```python
from build123d import *

# Parameters (mm, degrees)
SKETCH1_W                 = 2.116666666
SKETCH1_H                 = 3.175
SKETCH1_W_2               = 3.175
SKETCH1_H_2               = 2.116666666
SKETCH1_W_3               = 6.35
SKETCH1_H_3               = 37.666666667
SKETCH1_W_4               = 33.666666667
SKETCH1_H_4               = 6.35
BOSS_EXTRUDE1_DEPTH       = 3.175
SKETCH3_W                 = 3.175
SKETCH3_H                 = 3.175
SKETCH3_W_2               = 97.825
SKETCH3_H_2               = 109.825
BOSS_EXTRUDE2_DEPTH       = 3.175
MIRROR5_COPY_1_SKETCH_W   = 2.116666666
MIRROR5_COPY_1_SKETCH_H   = 3.175
MIRROR5_COPY_1_SKETCH_W_2 = 3.175
MIRROR5_COPY_1_SKETCH_H_2 = 2.116666666
MIRROR5_COPY_1_SKETCH_W_3 = 6.35
MIRROR5_COPY_1_SKETCH_H_3 = 37.666666667
MIRROR5_COPY_1_SKETCH_W_4 = 33.666666667
MIRROR5_COPY_1_SKETCH_H_4 = 6.35
MIRROR5_COPY_1_DEPTH      = 3.175
MIRROR5_COPY_2_SKETCH_W   = 3.175
MIRROR5_COPY_2_SKETCH_H   = 3.175
MIRROR5_COPY_2_SKETCH_W_2 = 97.825
MIRROR5_COPY_2_SKETCH_H_2 = 109.825
MIRROR5_COPY_2_DEPTH      = 3.175


with BuildPart() as part:
    # Sketch1 → Boss-Extrude1 (new body)
    # profile 1 of 4: a face of its own
    with BuildSketch(Plane(origin=(0, 0, 0), x_dir=(1, 0, 0), z_dir=(0, 1, 0))):
        Polygon((0, 122.525), (0, 135.225), (-123.225, 135.225), (-123.225, 0), (-110.525, 0), (-110.525, 37.666666667), (-110.525, 40.841666667), (-110.525, 122.525), (-78.927699489, 122.525), (-36.841666667, 122.525), (-33.666666667, 122.525), align=None)
        with Locations((-113.7, 39.254166667)):
            Rectangle(SKETCH1_W, SKETCH1_H, mode=Mode.SUBTRACT)
        with Locations((-35.254166667, 125.7)):
            Rectangle(SKETCH1_W_2, SKETCH1_H_2, mode=Mode.SUBTRACT)
    # profile 2 of 4: a face of its own
    with BuildSketch(Plane(origin=(0, 0, 0), x_dir=(1, 0, 0), z_dir=(0, 1, 0))):
        with Locations((-107.35, 18.833333334)):
            Rectangle(SKETCH1_W_3, SKETCH1_H_3)
    # profile 3 of 4: a face of its own
    with BuildSketch(Plane(origin=(0, 0, 0), x_dir=(1, 0, 0), z_dir=(0, 1, 0))):
        Polygon((-36.841666667, 113), (-36.841666667, 122.525), (-78.927699489, 122.525), (-110.525, 122.525), (-110.525, 40.841666667), (-101, 40.841666667), (-101, 113), align=None)
    # profile 4 of 4: a face of its own
    with BuildSketch(Plane(origin=(0, 0, 0), x_dir=(1, 0, 0), z_dir=(0, 1, 0))):
        with Locations((-16.833333334, 119.35)):
            Rectangle(SKETCH1_W_4, SKETCH1_H_4)
    boss_extrude1 = extrude(amount=BOSS_EXTRUDE1_DEPTH)

    # Sketch3 → Boss-Extrude2 (add)
    with BuildSketch(Plane(origin=(0, 3.175, 0), x_dir=(1, 0, 0), z_dir=(0, 1, 0))):
        with Locations((-99.4125, 111.4125)):
            Rectangle(SKETCH3_W, SKETCH3_H)
        with Locations((-48.9125, 111.4125)):
            Rectangle(SKETCH3_W_2, SKETCH3_H)
        with Locations((-99.4125, 54.9125)):
            Rectangle(SKETCH3_W, SKETCH3_H_2)
    boss_extrude2 = extrude(amount=-BOSS_EXTRUDE2_DEPTH)

    # Mirror4: Boss-Extrude1, Boss-Extrude2 across plane
    add(boss_extrude1.mirror(Plane(origin=(0, 0, 0), x_dir=(0, 0, 1), z_dir=(1, 0, 0))))
    add(boss_extrude2.mirror(Plane(origin=(0, 0, 0), x_dir=(0, 0, 1), z_dir=(1, 0, 0))))

    # Mirror5: Boss-Extrude1, Boss-Extrude2 across plane
    add(boss_extrude1.mirror(Plane.XY))
    add(boss_extrude2.mirror(Plane.XY))

    # Mirror5 copy 1 sketch → Mirror5 copy 1 (add)
    # profile 1 of 4: a face of its own
    with BuildSketch(Plane(origin=(0, 0, 0), x_dir=(-1, 0, 0), z_dir=(0, 1, 0))):
        Polygon((0, 122.525), (0, 135.225), (-123.225, 135.225), (-123.225, 0), (-110.525, 0), (-110.525, 37.666666667), (-110.525, 40.841666667), (-110.525, 122.525), (-78.927699489, 122.525), (-36.841666667, 122.525), (-33.666666667, 122.525), align=None)
        with Locations((-113.7, 39.254166667)):
            Rectangle(MIRROR5_COPY_1_SKETCH_W, MIRROR5_COPY_1_SKETCH_H, mode=Mode.SUBTRACT)
        with Locations((-35.254166667, 125.7)):
            Rectangle(MIRROR5_COPY_1_SKETCH_W_2, MIRROR5_COPY_1_SKETCH_H_2, mode=Mode.SUBTRACT)
    # profile 2 of 4: a face of its own
    with BuildSketch(Plane(origin=(0, 0, 0), x_dir=(-1, 0, 0), z_dir=(0, 1, 0))):
        with Locations((-107.35, 18.833333334)):
            Rectangle(MIRROR5_COPY_1_SKETCH_W_3, MIRROR5_COPY_1_SKETCH_H_3)
    # profile 3 of 4: a face of its own
    with BuildSketch(Plane(origin=(0, 0, 0), x_dir=(-1, 0, 0), z_dir=(0, 1, 0))):
        Polygon((-36.841666667, 113), (-36.841666667, 122.525), (-78.927699489, 122.525), (-110.525, 122.525), (-110.525, 40.841666667), (-101, 40.841666667), (-101, 113), align=None)
    # profile 4 of 4: a face of its own
    with BuildSketch(Plane(origin=(0, 0, 0), x_dir=(-1, 0, 0), z_dir=(0, 1, 0))):
        with Locations((-16.833333334, 119.35)):
            Rectangle(MIRROR5_COPY_1_SKETCH_W_4, MIRROR5_COPY_1_SKETCH_H_4)
    extrude(amount=MIRROR5_COPY_1_DEPTH)

    # Mirror5 copy 2 sketch → Mirror5 copy 2 (add)
    with BuildSketch(Plane(origin=(0, 3.175, 0), x_dir=(-1, 0, 0), z_dir=(0, 1, 0))):
        with Locations((-99.4125, 111.4125)):
            Rectangle(MIRROR5_COPY_2_SKETCH_W, MIRROR5_COPY_2_SKETCH_H)
        with Locations((-48.9125, 111.4125)):
            Rectangle(MIRROR5_COPY_2_SKETCH_W_2, MIRROR5_COPY_2_SKETCH_H)
        with Locations((-99.4125, 54.9125)):
            Rectangle(MIRROR5_COPY_2_SKETCH_W, MIRROR5_COPY_2_SKETCH_H_2)
    extrude(amount=-MIRROR5_COPY_2_DEPTH)


solid = part.part
```
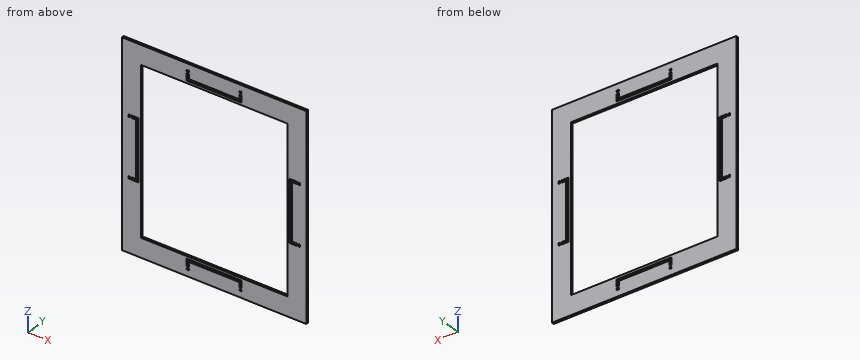
Verification items for the finished model (mm, model axes). Give positions to 0.01 mm unless a question says otherwise; leave off trailing zeros. Loops run counter-clockwise (first coordinate to the right, second up) from the corner with the lowest first, then second, coordinate; pieces in that order, holes last.
1. Section check C-C, the plane x = -78. Enter the section's corners in (y, z) (3 decimals), then the cut area to 3 significant figures.
2. Thickness scan on line 1 (X direction, y = 1, z = 11) (3 decimals); line 2 (Z direction, x = 12, y = 2.05) (3 decimals); line 3 (Z direction, x = -105.5, y = 1.3) (3 decimals). Record the ranges inside material, lowest first.
3. Section check B-B, the plane x = 17.5. Enter the section's corners in (y, z) (3 decimals), then the cut area to 3 significant figures.
4. Section check D-D, the plane y = 1.65. Count the separate pieces of the cut face and the enclosed holes in it, then the cut area to 3 significant figures.
5. Section check A-A, the plane z = -90. Enter the section's corners in (x, y) (3 decimals).
Geometry says:
1. outline: (0, -135.225) - (3.175, -135.225) - (3.175, -109.825) - (0, -109.825) - close; (0, 109.825) - (3.175, 109.825) - (3.175, 135.225) - (0, 135.225) - close
1. area: 161 mm2
2. line 1: x = -123.225 to -104.175, -101 to -97.825, 97.825 to 101, 104.175 to 123.225
2. line 2: z = -135.225 to -116.175, -113 to -109.825, 109.825 to 113, 116.175 to 135.225
2. line 3: z = -135.225 to -40.842, -37.667 to 37.667, 40.842 to 135.225
3. outline: (0, -135.225) - (3.175, -135.225) - (3.175, -116.175) - (0, -116.175) - close; (0, -113) - (3.175, -113) - (3.175, -109.825) - (0, -109.825) - close; (0, 109.825) - (3.175, 109.825) - (3.175, 113) - (0, 113) - close; (0, 116.175) - (3.175, 116.175) - (3.175, 135.225) - (0, 135.225) - close
3. area: 141 mm2
4. separate pieces: 1
4. enclosed holes: 13
4. area: 22,500 mm2
5. outline: (-123.225, 0) - (-97.825, 0) - (-97.825, 3.175) - (-123.225, 3.175) - close; (97.825, 0) - (123.225, 0) - (123.225, 3.175) - (97.825, 3.175) - close
